Check sheet for the drawn part. Datum: minimum x, y, z corner. Units: mm. A direction names the side the tool comes from. Round coordinates to 2 decimals unless told otherwise and drop trailing zeros. Order: outer loops, then holes, each group sorted by start corner. A loop starts at its lowest first (then second) coordinate and runs counter-clockwise, first axis right, second up.
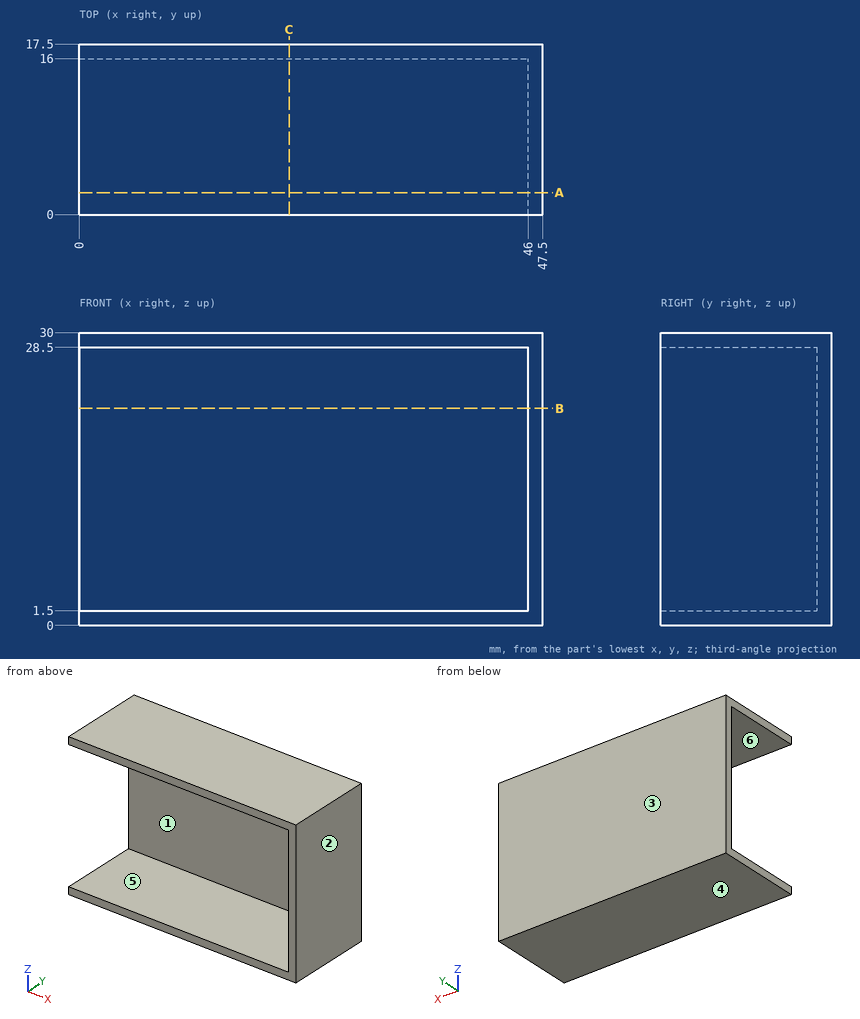
(1) Set-up check for the marked faces 1 and 2: record each of +Z, -Z, +X, -X, +Y, -Y from which the full face is reachable in a straight line by a thin tool's end or side.
Returned:
face 1: -X, -Y
face 2: +Z, -Z, +X, +Y, -Y
(2) Material ranges on line 1 (Z direction, x = 25.5, y = 15.25); line 2 (X direction, y = 11, z = 15.75); line 3 (Y direction, x = 27, z = 25.5), recorded low to high.
Returned:
line 1: z = 0 to 1.5, 28.5 to 30
line 2: x = 46 to 47.5
line 3: y = 16 to 17.5
(3) Sectioned sample at A-A, the plane y = 2.25. Record the cut outline in (x, z).
Returned:
outline: (0, 0) - (47.5, 0) - (47.5, 30) - (0, 30) - (0, 28.5) - (46, 28.5) - (46, 1.5) - (0, 1.5) - close
(4) Depth check by flat-ended pin: P1, Ø13.5, axis at x = 23, z = 11.5, coming from the -Y side. Enter the tip coordinate at first touch or a pass-through.
Returned:
P1: stops at y = 16
(5) Sectioned sample at C-C, the plane x = 21.5. Record the cut outline in (y, z), and give its area (3 significant figures).
Returned:
outline: (0, 0) - (17.5, 0) - (17.5, 30) - (0, 30) - (0, 28.5) - (16, 28.5) - (16, 1.5) - (0, 1.5) - close
area: 93.0 mm2
(6) Sectioned sample at B-B, the plane z = 22.25. Record the cut outline in (x, y).
Returned:
outline: (0, 16) - (46, 16) - (46, 0) - (47.5, 0) - (47.5, 17.5) - (0, 17.5) - close
(7) Draft check along Z on the marked faces 3, 4, 5 and 6. Enter one of: released by +Z, released by -Z, zero draft, split by the parting line, or undercut.
Returned:
face 3: zero draft
face 4: released by -Z
face 5: undercut
face 6: undercut
